For this review, take the finished solid that the model builds, in its own axes (mm). Coordinates: 2 decimals unless noted, no trailing zeros. Loops run counter-clockwise (first coordinate to the right, second up) from the corner with the lowest first, then second, coordinate; pieces in that order, holes last. Notation, with made-up numbers: M 80.5,79.25 L 95.5,79.25 A10 cw 95.5,97.25 Z; hole C 46.25,32.5 d8. An arc over 180 degrees is marked long. Write item = value, one per line.
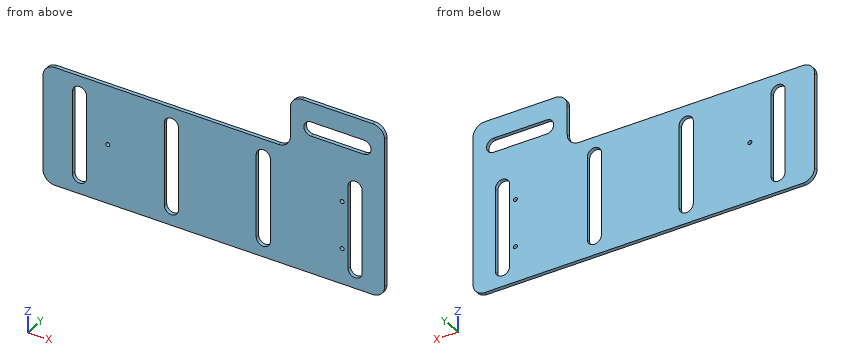
from build123d import *

# Parameters (mm, degrees)
BOSS_EXTRUDE1_DEPTH = 3.175
FILLET1_R           = 10
STANDOFF_HOLES_D    = 3.4
CUT_EXTRUDE1_DEPTH  = 3.175


with BuildPart() as part:
    # Sketch1 → Boss-Extrude1 (new body)
    with BuildSketch(Plane(origin=(0, 0, 0), x_dir=(1, 0, 0), z_dir=(0, 1, 0))):
        Polygon((-37.5, -50), (-145, -50), (-145, 50), (145, 50), (145, -50), (145, -95), (65, -95), (65, -50), (37.5, -50), align=None)
    extrude(amount=BOSS_EXTRUDE1_DEPTH)

    # Fillet1
    fillet1_edges = [part.edges().sort_by_distance(p)[0] for p in [
        (-145, 1.5875, 50),
        (-145, 1.5875, -50),
        (145, 1.5875, -50),
        (145, 1.5875, 95),
        (65, 1.5875, 95),
        (65, 1.5875, 50),
    ]]
    fillet(fillet1_edges, radius=FILLET1_R)

    # standoff holes (through all)
    with Locations(Plane(origin=(0, 3.175, 0), x_dir=(1, 0, 0), z_dir=(0, 1, 0))):
        with Locations((-90, 0), (109, 20), (109, -20)):
            Hole(STANDOFF_HOLES_D / 2)

    # Sketch6 → Cut-Extrude1 (cut)
    with BuildSketch(Plane(origin=(0, 3.175, 0), x_dir=(1, 0, 0), z_dir=(0, 1, 0))):
        with BuildLine():
            Line((-108, 35), (-108, -35))
            ThreePointArc((-108, -35), (-114, -41), (-120, -35))
            Line((-120, -35), (-120, 35))
            ThreePointArc((-120, 35), (-114, 41), (-108, 35))
        make_face()
        with BuildLine():
            Line((-30, 35), (-30, -35))
            ThreePointArc((-30, -35), (-36, -41), (-42, -35))
            Line((-42, -35), (-42, 35))
            ThreePointArc((-42, 35), (-36, 41), (-30, 35))
        make_face()
        with BuildLine():
            Line((48, 35), (48, -35))
            ThreePointArc((48, -35), (42, -41), (36, -35))
            Line((36, -35), (36, 35))
            ThreePointArc((36, 35), (42, 41), (48, 35))
        make_face()
        with BuildLine():
            Line((126, 35), (126, -35))
            ThreePointArc((126, -35), (120, -41), (114, -35))
            Line((114, -35), (114, 35))
            ThreePointArc((114, 35), (120, 41), (126, 35))
        make_face()
        with BuildLine():
            Line((82.5, -66.5), (127.5, -66.5))
            ThreePointArc((127.5, -66.5), (133.5, -72.5), (127.5, -78.5))
            Line((127.5, -78.5), (82.5, -78.5))
            ThreePointArc((82.5, -78.5), (76.5, -72.5), (82.5, -66.5))
        make_face()
    extrude(amount=-CUT_EXTRUDE1_DEPTH, mode=Mode.SUBTRACT)


solid = part.part
Q1. Add section B-B (z = 72.5). Write out the cut boundary in (x, y) (3 decimals), and give its area (3 significant figures).
Solved:
outline = M 65,0 L 76.5,0 L 76.5,3.175 L 65,3.175 Z; M 133.5,0 L 145,0 L 145,3.175 L 133.5,3.175 Z
area = 73.0 mm²
Q2. For line 1 along Z through (x, y) = (109, 1.6); line 2 along X through (y, z) = (2.85, -9); line 3 along X through (y, z) = (2.2, 20), list the stretches that pass through material, from the lowest coordinate up.
Solved:
line_1 = -50 to -21.7, -18.3 to 18.3, 21.7 to 66.5, 78.5 to 95
line_2 = -145 to -120, -108 to -42, -30 to 36, 48 to 114, 126 to 145
line_3 = -145 to -120, -108 to -42, -30 to 36, 48 to 107.3, 110.7 to 114, 126 to 145
Q3. Add section A-A (x = -114). Write out the cut boundary in (y, z) (3 decimals), and give its area (4 significant figures).
Solved:
outline = M 0,-50 L 3.175,-50 L 3.175,-41 L 0,-41 Z; M 0,41 L 3.175,41 L 3.175,50 L 0,50 Z
area = 57.15 mm²
Q4. Add section C-C (x = 120). Write out the cut boundary in (y, z) (3 decimals).
Solved:
outline = M 0,-50 L 3.175,-50 L 3.175,-41 L 0,-41 Z; M 0,41 L 3.175,41 L 3.175,66.5 L 0,66.5 Z; M 0,78.5 L 3.175,78.5 L 3.175,95 L 0,95 Z
Q5. Add section D-D (y = 2.3). State how many separate pieces and enclosed holes the cut face has, and give its area (3 significant figures).
Solved:
separate_pieces = 1
enclosed_holes = 8
area = 28,000 mm²
Q6. For pin 1 Ø1.6 at (y, z) = (1, 67.5) entering from -X; pin 2 Ø2.5 at (x, z) = (109, 20) entering from +Y; pin 3 Ø1.6 at (x, y) = (4.5, 2) entering from +Z, all flat-tipped, find the tip position at first contact; note any pin that passes through.
Solved:
pin_1 = 65
pin_2 = through
pin_3 = 50
